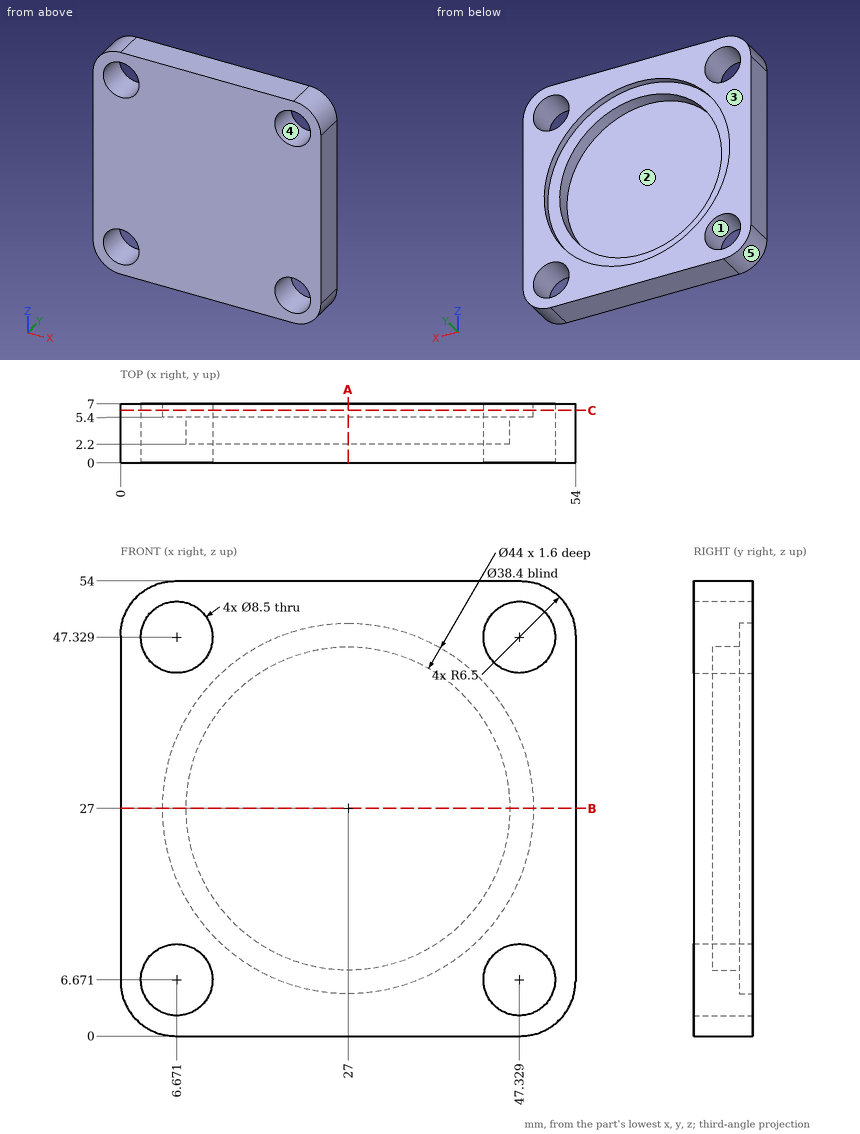
Could you check a few things on this drawing? It's one solid part, dimensions in mm from its lowest x, y, z. A direction names the side the tool comes from. Coordinates: 2 decimals unless noted, no trailing zeros. Order: outer loops, then holes, each group sorted by start corner. A loop starts at its lowest first (then second) coordinate and runs counter-clockwise, first axis right, second up. Notation, with made-up numbers: M 27,-4 L 68,-4 A11 ccw 68,3 Z; hole C -26,75.25 d6. An arc over 180 degrees is marked long. Answer as a JSON object with one key per item and string values. Group by question number.
(1) If we mould it in two halves opening along X, with no side actions, what happens to the marked faces 3, 4 and 5? For each: released by +X, released by -X, zero draft, split by the parting line, or undercut.
(2) Suppose I cut it at A-A, the plane x = 27. Please give me the cut outline in (y, z).
(3) Suppose I cut it at C-C, the plane y = 6.25. Please give me the cut outline in (x, z), then the cut area to 3 significant figures.
(4) Suppose I cut it at B-B, the plane z = 27. Please give me the cut outline in (x, y).
(5) I need wall thicknesses on probe 1 along X at (y, z) = (5, 6.5); probe 2 along Z at (x, y) = (47, 3.5); probe 3 along X at (y, z) = (6, 27). Which ranges of each line are inside material? Lowest first, please.
(6) Which directions (+Z, -Z, +X, -X, +Y, -Y) give clear straight access to the entire face, cutting with the end or side of a thin tool? Please do the marked faces 1 and 2.
(7) For pin 1 (13.5 mm diameter, centred on x = 6.67, z = 47.33, fed in from -Y); pin 2 (22 mm diameter, centred on x = 32, z = 28, fed in from +Y), each with a flat end and sliding along its axis, tell me the tip position at first contact or that it passes through.
Values found:
{
 "1": {"face 3": "zero draft", "face 4": "undercut", "face 5": "released by -X"},
 "2": {"outline": "M 0,0 L 7,0 L 7,5 L 5.4,5 L 5.4,7.8 L 2.2,7.8 L 2.2,46.2 L 5.4,46.2 L 5.4,49 L 7,49 L 7,54 L 0,54 Z"},
 "3": {"outline": "M 0,6.5 A6.5 ccw 6.5,0 L 47.5,0 A6.5 ccw 54,6.5 L 54,47.5 A6.5 ccw 47.5,54 L 6.5,54 A6.5 ccw 0,47.5 Z; hole C 6.67,6.67 d8.5; hole C 6.67,47.33 d8.5; hole C 27,27 d44; hole C 47.33,6.67 d8.5; hole C 47.33,47.33 d8.5", "area": "1,130 mm^2"},
 "4": {"outline": "M 0,0 L 54,0 L 54,7 L 49,7 L 49,5.4 L 46.2,5.4 L 46.2,2.2 L 7.8,2.2 L 7.8,5.4 L 5,5.4 L 5,7 L 0,7 Z"},
 "5": {"probe 1": "x = 0 to 2.42, 10.92 to 43.08, 51.58 to 54", "probe 2": "z = 0 to 2.43, 10.91 to 43.09, 51.57 to 54", "probe 3": "x = 0 to 5, 49 to 54"},
 "6": {"face 1": "+Y, -Y", "face 2": "+Y"},
 "7": {"pin 1": "stops at y = 0", "pin 2": "stops at y = 2.2"}
}
